Autodesk Inventor part; units mm, degrees
ref_plane "Work Plane1" through (0, 0, 170) normal (0, 0, 1) x (1, 0, 0)
ref_plane "Work Plane2" through (0, 0, 100) normal (0, 0, 1) x (1, 0, 0)
ref_plane "YZ Plane" through (0, 0, 0) normal (1, 0, 0) x (0, 1, 0)
sketch "Sketch1" plane through (0, 0, 0) normal (0, 0, 1) x (1, 0, 0)
  line L0 (0, 0) -> (-20, 0)
  line L1 (-20, 0) -> (-20, 10)
  line L2 (-20, 10) -> (0, 10)
  line L3 (0, 10) -> (0, 0)
  line L4 (-10, 0) -> (24.641, 0) construction
  line L5 (-10, 0) -> (24.641, 0) construction
  line L6 (0, 10) -> (20, 10)
  line L7 (20, 10) -> (20, -10)
  line L8 (-20, 10) -> (-40, 10)
  line L9 (-40, 10) -> (-40, -10)
  arc A0 (20, -10) -> (-40, -10) centre (-10, -48.9954) ccw
  point P0 (-5.5176, 0)
  point P1 (-14.4824, 0)
  dimension "d0" = 20
  dimension "d1" = 10
  dimension "d8" = 30
  dimension "d10" = 30
  dimension "d15" = 20
  dimension "d16" = 20
extrude "Extrusion1" add sketch "Sketch1" along normal blind 200
sketch "Sketch4" plane through (-40, 10, 0) normal (0, 1, 0) x (1, 0, 0)
  line L0 (0, 0) -> (0, -200)
  line L1 (60, 0) -> (60, -200)
  line L2 (0, 0) -> (60, -200) construction
  circle A0 centre (30, -100) radius 2
  point P0 (40, 0)
  dimension "d17" = 4
extrude "Extrusion4" cut sketch "Sketch4" against normal through all
ref_plane "Work Plane1" through (0, 0, 170) normal (0, 0, 1) x (1, 0, 0)
sketch "Sketch5" plane through (0, 0, 200) normal (0, 0, 1) x (1, 0, 0)
  line L0 (20, 10) -> (-40, 10)
  line L1 (-10, 10) -> (-40, 4)
  line L2 (-10, 10) -> (-40, 10)
  line L3 (-40, 4) -> (-40, 10)
  line L4 (-10, 10) -> (-10, 14.555) construction
  line L5 (-40, 10) -> (20, 10)
  line L6 (-10, 10) -> (20, 4)
  line L7 (-10, 10) -> (20, 10)
  line L8 (20, 4) -> (20, 10)
  line L9 (-15, 9) -> (-5, 9)
  point P0 (0, 0)
  dimension "d21" = 6
  dimension "d24" = 1
extrude "Extrusion5" cut sketch "Sketch5" against normal blind 10 from surface at -30
ref_plane "Work Plane2" through (0, 0, 100) normal (0, 0, 1) x (1, 0, 0)
mirror "Mirror1" about plane through (0, 0, 100) normal (0, 0, 1) of "Extrusion5"
equation "\"d10\" = d8"
equation "\"d16\" = d15"
properties part number "legno 2" material "Wood (Birch)"
The listing builds one solid part. Answer for the finished solid, in the listing's coordinates (mm). A direction names the side the tool comes from. Coordinates: 2 decimals unless noted, no trailing zeros. Loops run counter-clockwise (first coordinate to the right, second up) from the corner with the lowest first, then second, coordinate; pieces in that order, holes last. Notation, with made-up numbers: (8, 32) -> (40, 32) arc R22 ccw to (40, 54) -> close; hole circle Ø4 at (-0.75, -28). An arc over 180 degrees is marked (long way). Use one line per item in the form item = value. Start each with the question number.
Item 1: The part is cut by section B-B on y = 6. Determine the outline of the cut face in (x, z), then the cut area to 3 significant figures.
Item 2: The part is cut by section D-D on z = 34.5. Determine the outline of the cut face in (x, y).
Item 3: Consider L1, parallel to Z at x = -10, y = 3; L2, parallel to X at y = 8, z = 100; L3, parallel to Y at x = -11, z = 122. Determine where each line is inside the solid, lowest interval first. Write a range as [from, to].
Item 4: A tool of negligible diameter and unlimited length cuts with its end or side. For faces 1 (the face through (-8, 0, 99)), 2 (the face through (-27.325, 6.535, 165.07)), 3 (the face through (-10.4, 9.7, 160)), 4 (the face through (7.675, 6.465, 34.93)), from which of +Z, -Z, +X, -X, +Y, -Y can it reach the whole face along a straight path? Write none if from no direction.
Item 5: Flat-ended cylindrical pins translate along their axes: pin 1 Ø3.5 at (x, z) = (-10, 100) entering from -Y; pin 2 Ø6 at (x, z) = (-25, 175) entering from -Y; pin 3 Ø1 at (x, z) = (2, 43) entering from -Y; pin 4 Ø4.5 at (x, z) = (-10.5, 128.5) entering from -Y. Find the tip coordinate at first contact, or state that the pin passes through.
Item 6: The part is cut by section A-A on x = -10. Determine the outline of the cut face in (y, z), then the cut area to 3 significant figures.
Item 7: The mould has two halves that part along Z. Classify faces 5 (the face through (-10, 10, 185)), 6 (the face through (-10, 2, 0)), 7 (the face through (-10, 5, 98)): released by +Z, released by -Z, zero draft, split by the parting line, or undercut.
Item 8: The part is cut by section C-C on y = -4.5. Determine the outline of the cut face in (x, z).
Answer key:
q1.outline = (-40, 0) -> (20, 0) -> (20, 30) -> (10, 30) -> (10, 40) -> (20, 40) -> (20, 160) -> (10, 160) -> (10, 170) -> (20, 170) -> (20, 200) -> (-40, 200) -> (-40, 170) -> (-30, 170) -> (-30, 160) -> (-40, 160) -> (-40, 40) -> (-30, 40) -> (-30, 30) -> (-40, 30) -> close; hole circle Ø4 at (-10, 100)
q1.area = 11,600 mm2
q2.outline = (-40, -10) arc R49.2 cw to (-14.48, 0) -> (-5.52, 0) arc R49.2 cw to (20, -10) -> (20, 4) -> (-5, 9) -> (-15, 9) -> (-40, 4) -> close
q3.L1 = [0, 98], [102, 200]
q3.L2 = [-40, -12], [-8, 20]
q3.L3 = [0, 10]
q4.face_1 = +Z, -Z, -Y
q4.face_2 = -X, +Y
q4.face_3 = +Y
q4.face_4 = +X, +Y
q5.pin_1 = through
q5.pin_2 = -3.21
q5.pin_3 = -1.41
q5.pin_4 = 0
q6.outline = (0, 0) -> (10, 0) -> (10, 30) -> (9, 30) -> (9, 40) -> (10, 40) -> (10, 98) -> (0, 98) -> close; (0, 102) -> (10, 102) -> (10, 160) -> (9, 160) -> (9, 170) -> (10, 170) -> (10, 200) -> (0, 200) -> close
q6.area = 1,940 mm2
q7.face_5 = zero draft
q7.face_6 = released by -Z
q7.face_7 = undercut
q8.outline = (-40, 0) -> (-31, 0) -> (-31, 200) -> (-40, 200) -> close; (11, 0) -> (20, 0) -> (20, 200) -> (11, 200) -> close
